Part model, mm, in its own coordinate system. A direction names the side the tool comes from. Coordinates: 2 decimals unless noted, no trailing zeros. Write each loop counter-clockwise with the first axis right and the second up, starting at its lowest first coordinate (ties: lowest second). Pieces come first, ordered by that corner, then holes. Notation, with made-up numbers: (61, 17.5) -> (105, 17.5) arc R18 ccw to (105, 26.5) -> close; hole circle Ø7 at (61.5, 79.25). An arc over 180 degrees is marked (long way). Write item = value, one per line. Start each with the question number.
Q1. Band-saw the part on C-C, the plane z = -80.5. List the corners of the cut face in (x, y).
Q2. Pin check, flat tips, straight feed: P1, Ø10, axis at x = 35.5, z = -41.5, coming from the +Y side; P2, Ø8, axis at x = -122, y = 96.5, coming from the +Z side; P3, Ø12, axis at y = 34.5, z = -14.5, coming from the -X side; P4, Ø4, axis at x = 36.5, y = -18.5, coming from the +Z side. Stop position of each tip, or through.
Q3. Tool access for faces 1 (the flat face through (-81, 99.715, -59)), 2 (the flat face through (-111.531, 105, -8)), 3 (the flat face through (-126.531, 118, -54)), 4 (the flat face through (33.42, -10.61, -59.3)): list every direction of +Z, -Z, +X, -X, +Y, -Y with a clear straight run to the whole face (end or side of a thin tool).
Q4. Band-saw the part on B-B, the plane x = 46.5. List the corners of the cut face in (y, z), plus the area to 3 significant figures.
Q5. Band-saw the part on D-D, the plane y = -24. List the corners of the cut face in (x, z), plus the area to 3 significant figures.
Q6. Pull direction Y, two halves, no side cores. Call faces 5 (the flat face through (-33.531, 105, -8)), 6 (the cylindrical face through (65.95, -54.67, -5.07)), 7 (the flat face through (1, 46.3, -59.3)), 8 (the flat face through (-86, 89.715, -59)): released by +Y, released by -Y, zero draft, split by the parting line, or undercut.
Q7. Band-saw the part on A-A, the plane z = -32. List the corners of the cut face in (x, y).
Q8. Probe line 1 (Z direction, x = 44.5, y = -25); line 2 (Y direction, x = -94.5, z = -79.5); line 3 (Y direction, x = -55, z = -9). List the from-to ranges inside material, lowest first.
from build123d import *

# Parameters (mm, degrees)
BOSS_EXTRU_1_DEPTH                  = 120
BOSS_EXTRU_3_DEPTH                  = 47.25
BOSS_EXTRU_4_DEPTH                  = 10
BOSS_EXTRU_5_DEPTH                  = 10
ESQUISSE6_W                         = 15
ESQUISSE6_H                         = 57.25
ENL_V_MAT_EXTRU_1_DEPTH             = 50
ESQUISSE7_W                         = 100
ESQUISSE7_H                         = 60
ENL_V_MAT_EXTRU_2_DEPTH             = 10
ESQUISSE8_R                         = 3.73
ENL_V_MAT_EXTRU_3_DEPTH             = 10
ENL_V_MAT_EXTRU_3_DIRECTION_2_REACH = 112


with BuildPart() as part:
    # Esquisse1 → Boss.-Extru.1 (new body)
    with BuildSketch(Plane.XY):
        Polygon((-33.531301397, 99.715192212), (69.079300245, -59.00488979), (62.817327254, -63.053179131), (-35.94556587, 89.715192212), (-136.531301397, 89.715192212), (-136.531301397, 99.715192212), align=None)
    extrude(amount=-BOSS_EXTRU_1_DEPTH)

    # Esquisse3 → Boss.-Extru.3 (add)
    with BuildSketch(Plane(origin=(0, 99.715192212, 0), x_dir=(1, 0, 0), z_dir=(0, 1, 0))):
        Polygon((-33.531301397, 110), (-33.531301397, 120), (-136.531301397, 120), (-136.531301397, 0), (-33.531301397, 0), (-33.531301397, 10), (-126.531301397, 10), (-126.531301397, 110), align=None)
    extrude(amount=BOSS_EXTRU_3_DEPTH)

    # Esquisse4 → Boss.-Extru.4 (add)
    with BuildSketch(Plane.XY):
        Polygon((-33.531301397, 146.965192212), (90.622108587, -45.077726339), (69.079300245, -59.00488979), (-33.531301397, 99.715192212), align=None)
    extrude(amount=-BOSS_EXTRU_4_DEPTH)

    # Esquisse5 → Boss.-Extru.5 (add)
    with BuildSketch(Plane(origin=(0, 0, -120), x_dir=(-1, 0, 0), z_dir=(0, 0, -1))):
        Polygon((33.531301397, 99.715192212), (33.531301397, 146.965192212), (-90.622108587, -45.077726339), (-69.079300245, -59.00488979), align=None)
    extrude(amount=-BOSS_EXTRU_5_DEPTH)

    # Esquisse6 → Enlèv. mat.-Extru.1 (cut)
    with BuildSketch(Plane.XY):
        with Locations((-119.031301397, 118.340192212)):
            Rectangle(ESQUISSE6_W, ESQUISSE6_H)
        with Locations((-41.031301397, 118.340192212)):
            Rectangle(ESQUISSE6_W, ESQUISSE6_H)
    extrude(amount=-ENL_V_MAT_EXTRU_1_DEPTH, mode=Mode.SUBTRACT)

    # Esquisse7 → Enlèv. mat.-Extru.2 (cut)
    with BuildSketch(Plane(origin=(21.815602094, 14.103521292, 0), x_dir=(0, 0, -1), z_dir=(0.839788794, 0.542913236, 0))):
        with Locations((60, -57.055711668)):
            Rectangle(ESQUISSE7_W, ESQUISSE7_H)
    extrude(amount=-ENL_V_MAT_EXTRU_2_DEPTH, mode=Mode.SUBTRACT)

    # Esquisse8 → Enlèv. mat.-Extru.3 (cut)
    with BuildSketch(Plane.XY.offset(-110)):
        with Locations((63.942262825, -57.813776091)):
            Circle(ESQUISSE8_R)
    extrude(amount=-ENL_V_MAT_EXTRU_3_DEPTH, mode=Mode.SUBTRACT)

    # Esquisse8 → Enlèv. mat.-Extru.3 direction 2 (cut, up to next)
    with BuildSketch(Plane.XY.offset(-110), mode=Mode.PRIVATE) as enl_v_mat_extru_3_direction_2_sk1:
        with Locations((63.942262825, -57.813776091)):
            Circle(ESQUISSE8_R)
    enl_v_mat_extru_3_direction_2_tool1 = extrude(enl_v_mat_extru_3_direction_2_sk1.sketch, amount=ENL_V_MAT_EXTRU_3_DIRECTION_2_REACH, mode=Mode.PRIVATE) & part.part
    add(enl_v_mat_extru_3_direction_2_tool1.solids().sort_by_distance((63.942263, -57.813776, -110))[0], mode=Mode.SUBTRACT)


solid = part.part
Ans:
q1.outline = (-136.53, 89.72) -> (-35.95, 89.72) -> (30.24, -12.67) -> (36.5, -8.62) -> (-33.53, 99.72) -> (-126.53, 99.72) -> (-126.53, 146.97) -> (-136.53, 146.97) -> close
q2.P1 = 0.67
q2.P2 = -50
q2.P3 = -4.13
q2.P4 = 0
q3.face_1 = +X, +Y
q3.face_2 = +Z, +Y, -Y
q3.face_3 = +Z, +Y
q3.face_4 = +X, -Y
q4.outline = (-37.81, -120) -> (23.17, -120) -> (23.17, -110) -> (-37.81, -110) -> close; (-37.81, -10) -> (23.17, -10) -> (23.17, 0) -> (-37.81, 0) -> close
q4.area = 1,220 mm2
q5.outline = (37.57, -120) -> (77, -120) -> (77, -110) -> (37.57, -110) -> close; (37.57, -10) -> (77, -10) -> (77, 0) -> (37.57, 0) -> close
q5.area = 789 mm2
q6.face_5 = zero draft
q6.face_6 = undercut
q6.face_7 = released by +Y
q6.face_8 = released by -Y
q7.outline = (-136.53, 89.72) -> (-126.53, 89.72) -> (-126.53, 146.97) -> (-136.53, 146.97) -> close; (-111.53, 89.72) -> (-48.53, 89.72) -> (-48.53, 99.72) -> (-111.53, 99.72) -> close; (-35.95, 89.72) -> (30.24, -12.67) -> (36.5, -8.62) -> (-33.53, 99.72) -> (-33.53, 89.72) -> close
q8.line_1 = -120 to -110, -10 to 0
q8.line_2 = 89.72 to 99.72
q8.line_3 = 89.72 to 146.97
